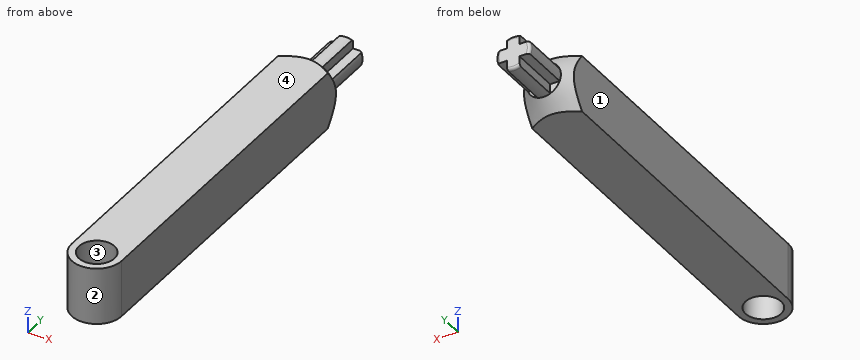
```python
from build123d import *

# Parameters (mm, degrees)
SKETCH_1_R      = 2.5
EXTRUDE_1_DEPTH = 8
EXTRUDE_3_DEPTH = 7
FILLET_1_R      = 0.4


with BuildPart() as part:
    # ｽｹｯﾁ1 → ﾎﾞｽ - 押し出し1 (new body)
    with BuildSketch(Plane.XY):
        with BuildLine():
            Line((-3.5, 0), (-3.5, 50))
            Line((-3.5, 50), (3.5, 50))
            Line((3.5, 50), (3.5, 0))
            ThreePointArc((3.5, 0), (0, -3.5), (-3.5, 0))
        make_face()
        Circle(SKETCH_1_R, mode=Mode.SUBTRACT)
    extrude(amount=EXTRUDE_1_DEPTH)

    # ｽｹｯﾁ2 → ﾎﾞｽ - 押し出し3 (add)
    with BuildSketch(Plane(origin=(0, 50, 0), x_dir=(1, 0, 0), z_dir=(0, 1, 0))):
        with BuildLine():
            Line((-0.89, -1.781892699), (-0.89, -3.11))
            Line((-0.89, -3.11), (-2.218107301, -3.11))
            ThreePointArc((-2.218107301, -3.11), (-2.39, -4), (-2.218107301, -4.89))
            Line((-2.218107301, -4.89), (-0.89, -4.89))
            Line((-0.89, -4.89), (-0.89, -6.218107301))
            ThreePointArc((-0.89, -6.218107301), (0, -6.39), (0.89, -6.218107301))
            Line((0.89, -6.218107301), (0.89, -4.89))
            Line((0.89, -4.89), (2.218107301, -4.89))
            ThreePointArc((2.218107301, -4.89), (2.39, -4), (2.218107301, -3.11))
            Line((2.218107301, -3.11), (0.89, -3.11))
            Line((0.89, -3.11), (0.89, -1.781892699))
            ThreePointArc((0.89, -1.781892699), (0, -1.61), (-0.89, -1.781892699))
        make_face()
    extrude(amount=EXTRUDE_3_DEPTH)

    # ﾌｨﾚｯﾄ1
    fillet_1_edges = [part.edges().sort_by_distance(p)[0] for p in [
        (0, 57, 1.61),
        (-2.39, 57, 4),
        (0, 57, 6.39),
        (2.39, 57, 4),
    ]]
    fillet(fillet_1_edges, radius=FILLET_1_R)

    # ｽｹｯﾁ5 → ｶｯﾄ - 回転2 (revolve, cut)
    with BuildSketch(Plane(origin=(-1.982300885, 0, 1.734513274), x_dir=(0.6585046078685183, 0, 0.7525766947068778), z_dir=(-0.7525766947068777, 0, 0.6585046078685182)), mode=Mode.PRIVATE) as cut_revolve_2_sk:
        Polygon((0.620306779, 50), (-2.304766128, 47), (-2.304766128, 50), align=None)
    revolve(cut_revolve_2_sk.sketch.rotate(Axis((0, 57, 4), (0, -1, 0)), 19.323147236), axis=Axis((0, 57, 4), (0, -1, 0)), mode=Mode.SUBTRACT)


solid = part.part
```
Input: part model. Units: mm. Frame: model coordinates. Face numbers are marked on the shaded views. Coordinates: 2 decimals unless noted, no trailing zeros. Loops run counter-clockwise (first coordinate to the right, second up) from the corner with the lowest first, then second, coordinate; pieces in that order, holes last. Notation, with made-up numbers: M 26,5 L 39,5 A7 cw 39,11 Z; hole C -30,-8.75 d6. An arc over 180 degrees is marked long. One line per item, written item: value.
(1) Pin query (flat end, axial travel): pin 1 (4 mm diameter, centred on x = 1, z = 6, fed in from +Y); pin 2 (1.5 mm diameter, centred on x = 1.5, y = 53.5, fed in from +Z); pin 3 (1.1 mm diameter, centred on x = 1.5, y = 54, fed in from -Z); pin 4 (0.7 mm diameter, centred on x = -1.5, z = 5.5, fed in from +Y). Return the tip coordinate at first contact, or that it passes through.
Filled in:
pin 1: y = 57
pin 2: z = 6.27
pin 3: z = 3.11
pin 4: y = 50
(2) Pull-direction query (X, two-part tool) for the marked faces 1, 2, 3 and 4; classes: +X half, -X half, draft (parallel to the pull), parting line (faces both ways), or undercut.
Filled in:
face 1: -X half
face 2: parting line
face 3: undercut
face 4: draft
(3) Section B-B (z = 4). Output: boundary loops of the cut face in (x, y).
Filled in:
outline: M -3.5,0 A3.5 ccw 3.5,0 L 3.5,48.86 L 2.39,50 L 2.39,56.6 A0.4 ccw 1.99,57 L -1.99,57 A0.4 ccw -2.39,56.6 L -2.39,50 L -3.5,48.86 Z; hole C 0,0 d5
(4) Line query: line 1 along Y through (x, z) = (-0.75, 2.75); line 2 along Y through (x, z) = (-2, 3.5); line 3 along Y through (x, z) = (-2.75, 2.75). Output: solid intervals per line, ascending. Write a range as from..to.
Filled in:
line 1: -3.42..-2.38, 2.38..57
line 2: -2.87..-1.5, 1.5..56.99
line 3: -2.17..49.35
(5) Section A-A (x = 0). Output: boundary loops of the cut face in (y, z), and give its area (3 significant figures).
Filled in:
outline: M -3.5,0 L -2.5,0 L -2.5,8 L -3.5,8 Z; M 2.5,0 L 48.35,0 L 50,1.61 L 56.6,1.61 A0.4 ccw 57,2.01 L 57,5.99 A0.4 ccw 56.6,6.39 L 50,6.39 L 48.35,8 L 2.5,8 Z
area: 419 mm^2
